Autodesk Inventor part; units mm, degrees
ref_plane "YZ Plane" through (0, 0, 0) normal (1, 0, 0) x (0, 1, 0)
ref_plane "XZ Plane" through (0, 0, 0) normal (0, 1, 0) x (-1, 0, 0)
ref_plane "XY Plane" through (0, 0, 0) normal (0, 0, 1) x (1, 0, 0)
sketch "Esboço11" plane through (0, 0, 0) normal (0, 0, 1) x (1, 0, 0)
  line L0 (0, 0) -> (354, 0)
  line L1 (354, 0) -> (354, 254)
  line L2 (354, 254) -> (0, 254)
  line L3 (0, 254) -> (0, 0)
  line L4 (2, 252) -> (352, 252)
  line L5 (352, 252) -> (352, 2)
  line L6 (352, 2) -> (2, 2)
  line L7 (2, 2) -> (2, 252)
  dimension "d14" = 354
  dimension "d15" = 254
  dimension "d16" = 2
  dimension "d17" = 2
  dimension "d18" = 2
  dimension "d19" = 2
extrude "Extrusão3" add sketch "Esboço11" along normal blind 250
sketch "Esboço12" plane through (0, 0, 250) normal (0, 0, 1) x (1, 0, 0)
  line L0 (2, 2) -> (2, 252)
  line L1 (352, 2) -> (2, 2)
  line L2 (2, 252) -> (352, 252)
  line L3 (352, 252) -> (352, 2)
  line L4 (352, 2) -> (2, 2)
  line L5 (2, 2) -> (2, 252)
  point P0 (0, 0)
extrude "Extrusão4" add sketch "Esboço12" against normal blind 2
fillet "Arredondamento1" radius 2 4 edges at (177, 254, 250) (177, 2, 248) (354, 127, 250) (0, 127, 250)
properties part number "Caixa"
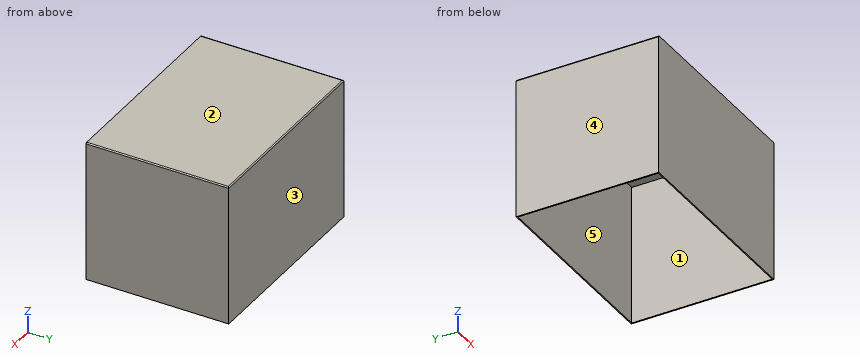
Input: part model. Units: mm. Frame: model coordinates. Face numbers are marked on the shaded views. A direction names the side the tool comes from. Coordinates: 2 decimals unless noted, no trailing zeros. Order: outer loops, then holes, each group sorted by start corner. A loop starts at its lowest first (then second) coordinate and runs counter-clockwise, first axis right, second up. Notation, with made-up numbers: M 32.25,68 L 70.25,68 A22 ccw 70.25,94 Z; hole C 71.5,44.25 d11. An arc over 180 degrees is marked long. Answer in a Markdown table with one row per item.
(1) Section query C-C, the plane x = 32. Output: boundary loops of the cut face in (y, z).
Numbers:
| item | result |
|---|---|
| outline | M 0,0 L 2,0 L 2,246 A2 cw 4,248 L 252,248 L 252,0 L 254,0 L 254,248 A2 ccw 252,250 L 0,250 Z |
(2) Material intervals for line 1 (Y direction, x = 262.5, z = 38); line 2 (X direction, y = 107.5, z = 181.5); line 3 (Z direction, x = 166, y = 158), sorted ascending. Write a range as [from, to].
Numbers:
| item | result |
|---|---|
| line 1 | y = [0, 2], [252, 254] |
| line 2 | x = [0, 2], [352, 354] |
| line 3 | z = [248, 250] |
(3) Section query B-B, the plane y = 118. Output: boundary loops of the cut face in (x, z), plus the area to 3 significant figures.
Numbers:
| item | result |
|---|---|
| outline | M 0,0 L 2,0 L 2,248 L 352,248 L 352,0 L 354,0 L 354,248 A2 ccw 352,250 L 2,250 A2 ccw 0,248 Z |
| area | 1,700 mm^2 |
(4) Section query A-A, the plane z = 218. Output: boundary loops of the cut face in (x, y), plus the area to 3 significant figures.
Numbers:
| item | result |
|---|---|
| outline | M 0,0 L 354,0 L 354,254 L 0,254 Z; hole M 2,2 L 352,2 L 352,252 L 2,252 Z |
| area | 2,420 mm^2 |
(5) Draft query along Y for the marked faces 3, 4 and 5. Return one class per face: pulls with the +Y half, pulls with the -Y half, needs draft (parallel to the pull), parting line crosses it, or undercut.
Numbers:
| item | result |
|---|---|
| face 3 | pulls with the +Y half |
| face 4 | needs draft |
| face 5 | undercut |
(6) Contact query for flat-ended pins moving along their axis: pin 1 Ø4 at (x, z) = (259.5, 198.5) entering from -Y; pin 2 Ø8 at (x, y) = (73, 138.5) entering from -Z. Output: stop coordinate, or through.
Numbers:
| item | result |
|---|---|
| pin 1 | stops at y = 0 |
| pin 2 | stops at z = 248 |
(7) Access query for the marked faces 1 and 2. Directions: +Z, -Z, +X, -X, +Y, -Y. A direction counts if a zero-diameter tool reaches every point of the face in a straight line with its end or side. Return the directions, or none.
Numbers:
| item | result |
|---|---|
| face 1 | -Z |
| face 2 | +Z, +X, -X, +Y, -Y |
